from build123d import *

# Parameters (mm, degrees)
SKETCH_1_W                 = 24
SKETCH_1_H                 = 24
EXTRUDE_1_DEPTH            = 4
SKETCH_6_R                 = 2
EXTRUDE_2_DEPTH            = 4
CHAMFER_1_SIZE             = 1
CHAMFER_1_OF_MIRROR_1_SIZE = 1


with BuildPart() as part:
    # Эскиз1 → Бобышка-Вытянуть1 (new body)
    # profile 1 of 5: a face of its own
    with BuildSketch(Plane.XY):
        Rectangle(SKETCH_1_W, SKETCH_1_H)
        Polygon((-3, 10), (0, 10), (3, 10), (5.5, 10), (10, 10), (10, 3), (10, -3), (10, -10), (3, -10), (-3, -10), (-10, -10), (-10, -3), (-10, 3), (-10, 10), (-5.5, 10), align=None, mode=Mode.SUBTRACT)
    # profile 2 of 5: a face of its own
    with BuildSketch(Plane.XY):
        Polygon((-3, -10), (3, -10), (3, -8.2), (5.5, -8.2), (5.5, -6.56), (3, -3.693992791), (-3, -3.693992791), (-5.5, -6.56), (-5.5, -8.2), (-3, -8.2), align=None)
    # profile 3 of 5: a face of its own
    with BuildSketch(Plane.XY):
        Polygon((10, -3), (10, 3), (8.2, 3), (8.2, 5.5), (6.56, 5.5), (3.693992791, 3), (3.693992791, -3), (6.56, -5.5), (8.2, -5.5), (8.2, -3), align=None)
    # profile 4 of 5: a face of its own
    with BuildSketch(Plane.XY):
        Polygon((-8.2, 3), (-10, 3), (-10, -3), (-8.2, -3), (-8.2, -5.5), (-6.56, -5.5), (-3.693992791, -3), (-3.693992791, 3), (-6.56, 5.5), (-8.2, 5.5), align=None)
    # profile 5 of 5: a face of its own
    with BuildSketch(Plane.XY):
        Polygon((3, 10), (0, 10), (-3, 10), (-3, 8.2), (-5.5, 8.2), (-5.5, 6.56), (-3, 3.693992791), (3, 3.693992791), (5.5, 6.56), (5.5, 8.2), (3, 8.2), align=None)
    extrude(amount=EXTRUDE_1_DEPTH)

    # Эскиз6 → Бобышка-Вытянуть2 (add)
    with BuildSketch(Plane(origin=(0, 12, 0), x_dir=(1, 0, 0), z_dir=(0, 1, 0))):
        with BuildLine():
            Line((-12, 2), (-18, 2))
            ThreePointArc((-18, 2), (-19.414213562, 1.414213562), (-20, 0))
            Line((-20, 0), (-20, -4))
            ThreePointArc((-20, -4), (-19.414213562, -5.414213562), (-18, -6))
            Line((-18, -6), (-12, -6))
            Line((-12, -6), (-12, 2))
        make_face()
        with Locations(Location((-16, -2, 0), (0, 0, 270))):
            Circle(SKETCH_6_R, mode=Mode.SUBTRACT)
    extrude_2 = extrude(amount=-EXTRUDE_2_DEPTH)

    # Фаска1
    chamfer_1_edges = [part.edges().sort_by_distance(p)[0] for p in [
        (-12, 10, -2),
        (-12, 10, 6),
    ]]
    chamfer(chamfer_1_edges, length=CHAMFER_1_SIZE)

    # Зеркальное отражение1: Бобышка-Вытянуть2 across plane
    add(extrude_2.mirror(Plane(origin=(0, 0, 0), x_dir=(0, 0, 1), z_dir=(1, 0, 0))))

    # Фаска1 of Зеркальное отражение1
    chamfer_1_of_mirror_1_edges = [part.edges().sort_by_distance(p)[0] for p in [
        (12, 10, -2),
        (12, 10, 6),
    ]]
    chamfer(chamfer_1_of_mirror_1_edges, length=CHAMFER_1_OF_MIRROR_1_SIZE)


solid = part.part
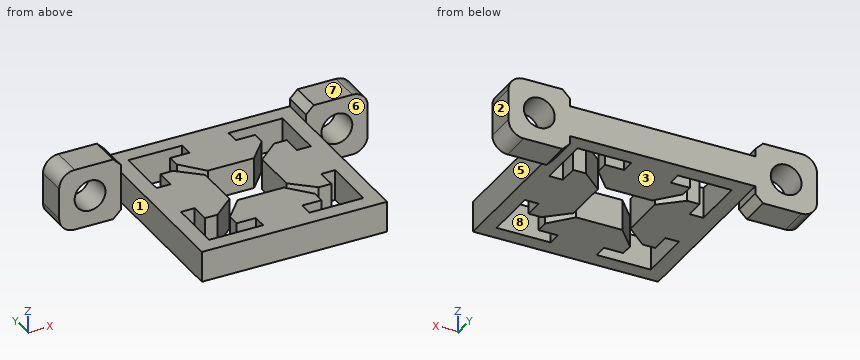
Can you work these out from the model? Positions are in its coordinate system, mm. Face numbers are marked on the shaded views. A direction names the side the tool comes from. Round coordinates to 2 decimals unless told otherwise and drop trailing zeros. Loops run counter-clockwise (first coordinate to the right, second up) from the corner with the lowest first, then second, coordinate; pieces in that order, holes last. Notation, with made-up numbers: (-20.5, 1) - (1.5, 1) arc R7 cw to (1.5, 12) - close; hole circle Ø10 at (-17.5, 49.25). An arc over 180 degrees is marked (long way). Answer in a Markdown table with one row per item. Add a question column.
Q1. I want a section at D-D on z = 2. Count the separate pieces of the cut face and the enclosed holes in it, and give its area (3 significant figures).
Q2. We'd pull the mould along Y, two halves only. Please class the marked faces 6, 7 and 8: pulls with the +Y half, pulls with the -Y half, needs draft (parallel to the pull), parting line crosses it, or undercut.
Q3. I want a section at A-A on y = 5. List the corners of the cut face in (x, z) for me, and give its area (3 significant figures).
Q4. I need wall thicknesses on L1, parallel to Y at x = 7.5, z = 1; L2, parallel to Y at x = -8.5, z = 3.5; L3, parallel to X at y = 9, z = 2. Which ranges of each line are inside material? Lowest first, please.
Q5. Which directions (+Z, -Z, +X, -X, +Y, -Y) give clear straight access to the entire face, cutting with the end or side of a thin tool? Please do the marked faces 1, 2, 3, 4 and 5.
Q6. For pin 1 Ø3 at (y, z) = (0, 1) entering from +X; pin 2 Ø4.5 at (y, z) = (0, 2) entering from -X; pin 3 Ø5 at (x, y) = (10, -7) entering from -Z, each with a flat end and sliding along its axis, tell me the tip position at first contact or that it passes through.
Q7. I want a section at B-B on x = -16. List the corners of the cut face in (y, z) for me.
Q8. I want a section at C-C on y = 2.5. List the corners of the cut face in (x, z) for me.
A:
| question | item | result |
|---|---|---|
| 1 | separate pieces | 3 |
| 1 | enclosed holes | 1 |
| 1 | area | 421 mm^2 |
| 2 | face 6 | pulls with the -Y half |
| 2 | face 7 | needs draft |
| 2 | face 8 | undercut |
| 3 | outline | (-12, 0) - (-10, 0) - (-10, 4) - (-12, 4) - close; (-8.2, 0) - (-5.99, 0) - (-5.99, 4) - (-8.2, 4) - close; (-4.14, 0) - (4.14, 0) - (4.14, 4) - (-4.14, 4) - close; (5.99, 0) - (8.2, 0) - (8.2, 4) - (5.99, 4) - close; (10, 0) - (12, 0) - (12, 4) - (10, 4) - close |
| 3 | area | 66.8 mm^2 |
| 4 | L1 | -12 to -10, -5.5 to 5.5, 10 to 12 |
| 4 | L2 | -12 to -10, -3 to 3, 10 to 12 |
| 4 | L3 | -20 to -18, -14 to -10, -3 to 3, 10 to 14, 18 to 20 |
| 5 | face 1 | +Z, -Z, -X, -Y |
| 5 | face 2 | +Z, -Z, +X, +Y, -Y |
| 5 | face 3 | -Z, +Y, -Y |
| 5 | face 4 | +Z, -Z |
| 5 | face 5 | +Z, -Z, +X, -Y |
| 6 | pin 1 | x = 12 |
| 6 | pin 2 | x = -12 |
| 6 | pin 3 | z = 0 |
| 7 | outline | (8, -2) - (12, -2) - (12, 0) - (8, 0) - close; (8, 4) - (12, 4) - (12, 6) - (8, 6) - close |
| 8 | outline | (-12, 0) - (-3.69, 0) - (-3.69, 4) - (-12, 4) - close; (3.69, 0) - (12, 0) - (12, 4) - (3.69, 4) - close |
